The listing builds one solid part. Answer for the finished solid, in the listing's coordinates (mm). Face numbers are marked on the shaded views. A direction names the side the tool comes from. Coordinates: 2 decimals unless noted, no trailing zeros. Order: outer loops, then holes, each group sorted by start corner. A loop starts at its lowest first (then second) coordinate and runs counter-clockwise, first axis right, second up. Notation, with made-up numbers: (-23, 61.25) -> (-15, 61.25) arc R22 ccw to (-15, 94.25) -> close; hole circle Ø8 at (31.25, 19). An arc over 180 degrees is marked (long way). Write each question's results on one line, items separated by ' | '. Start each with the question number.
(1) The part is cut by section B-B, the plane x = -7.5. Give the vertices of the cut face in (y, z), then the cut area to 3 significant figures.
(2) Determine the mould class of the marked faces 6, 7 and 8 for opening direction Z: +Z half, -Z half, draft (parallel to the pull), parting line (faces both ways), or undercut.
(3) A tool of negligible diameter and unlimited length cuts with its end or side. For the marked faces 1, 2, 3, 4 and 5, from which of +Z, -Z, +X, -X, +Y, -Y can it reach the whole face along a straight path? Write none if from no direction.
(4) The part is cut by section C-C, the plane y = 0.55. Give the vertices of the cut face in (x, z).
(5) Given pin 1 (4.5 mm diameter, centred on x = -7.5, z = -11.25, fed in from +Y); pin 2 (2.5 mm diameter, centred on x = -7.5, z = -3.75, fed in from +Y); pin 3 (3 mm diameter, centred on x = -1, z = -8, fed in from -Y); pin 4 (3.5 mm diameter, centred on x = -8.5, z = -5.5, fed in from -Y), each flat-ended and moving along its own axis, determine where each tip first touches the part or whether it passes through.
(6) The part is cut by section D-D, the plane x = -1.25. Give the vertices of the cut face in (y, z), then the cut area to 3 significant figures.
(7) Straight lines are drawn through the part: L1, parallel to Z at x = -0.5, y = 2.15; L2, parallel to X at y = 3.35, z = -7.5; L3, parallel to Z at x = -7, y = 0.5. For each, find the intervals that lie inside material, in ascending order.
(8) The part is cut by section A-A, the plane z = -11.25. Give the vertices of the cut face in (x, y).
```python
from build123d import *

# Parameters (mm, degrees)
SKETCH1_W           = 11
SKETCH1_H           = 15
BOSS_EXTRUDE3_DEPTH = 2
SKETCH2_W           = 4
SKETCH2_H           = 15
BOSS_EXTRUDE4_DEPTH = 2
SKETCH3_W           = 4
SKETCH3_H           = 15
BOSS_EXTRUDE5_DEPTH = 2
SKETCH4_R           = 1.65
CUT_EXTRUDE2_DEPTH  = 13
SKETCH6_W           = 11
SKETCH6_H           = 3
CUT_EXTRUDE4_DEPTH  = 3.8
SKETCH7_R           = 1.5
CUT_EXTRUDE5_DEPTH  = 17.8


with BuildPart() as part:
    # Sketch1 → Boss-Extrude3 (new body)
    with BuildSketch(Plane(origin=(0, 0, 0), x_dir=(1, 0, 0), z_dir=(0, 1, 0))):
        with Locations((-5.5, 7.5)):
            Rectangle(SKETCH1_W, SKETCH1_H)
    extrude(amount=BOSS_EXTRUDE3_DEPTH)

    # Sketch2 → Boss-Extrude4 (add)
    with BuildSketch(Plane(origin=(0, 2, 0), x_dir=(1, 0, 0), z_dir=(0, 1, 0))):
        with Locations((-2, 7.5)):
            Rectangle(SKETCH2_W, SKETCH2_H)
    extrude(amount=BOSS_EXTRUDE4_DEPTH)

    # Sketch3 → Boss-Extrude5 (add)
    with BuildSketch(Plane(origin=(0, 0, 0), x_dir=(-1, 0, 0), z_dir=(0, -1, 0))):
        with Locations((2, 7.5)):
            Rectangle(SKETCH3_W, SKETCH3_H)
    extrude(amount=BOSS_EXTRUDE5_DEPTH)

    # Sketch4 → Cut-Extrude2 (cut)
    with BuildSketch(Plane(origin=(0, 0, 0), x_dir=(-1, 0, 0), z_dir=(0, -1, 0))):
        with Locations(Location((7.5, 11.25, 0), (0, 0, 90))):
            Circle(SKETCH4_R)
        with Locations(Location((7.5, 3.75, 0), (0, 0, 90))):
            Circle(SKETCH4_R)
    extrude(amount=-CUT_EXTRUDE2_DEPTH, mode=Mode.SUBTRACT)

    # Sketch6 → Cut-Extrude4 (cut)
    with BuildSketch(Plane(origin=(0, 0, 0), x_dir=(0, 0, -1), z_dir=(1, 0, 0))):
        with Locations((7.5, 1)):
            Rectangle(SKETCH6_W, SKETCH6_H)
    extrude(amount=-CUT_EXTRUDE4_DEPTH, mode=Mode.SUBTRACT)

    # Sketch7 → Cut-Extrude5 (cut)
    with BuildSketch(Plane(origin=(0, -2, 0), x_dir=(-1, 0, 0), z_dir=(0, -1, 0))):
        with Locations(Location((2, 7.5, 0), (0, 0, 90))):
            Circle(SKETCH7_R)
    extrude(amount=-CUT_EXTRUDE5_DEPTH, mode=Mode.SUBTRACT)


solid = part.part
```
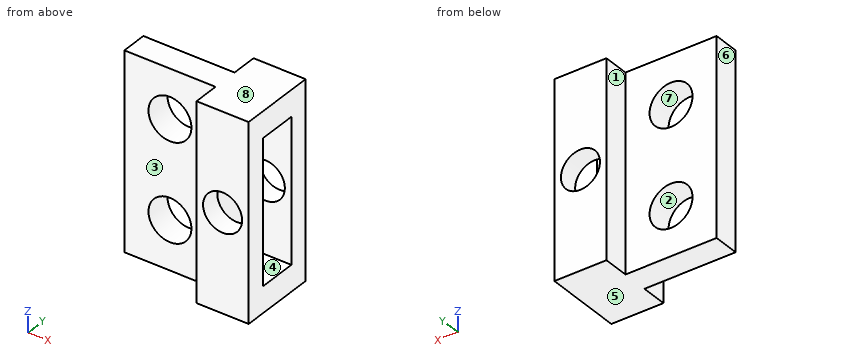
Established:
1) outline: (0, -15) -> (2, -15) -> (2, -12.9) -> (0, -12.9) -> close; (0, -9.6) -> (2, -9.6) -> (2, -5.4) -> (0, -5.4) -> close; (0, -2.1) -> (2, -2.1) -> (2, 0) -> (0, 0) -> close | area: 16.8 mm^2
2) face 6: draft | face 7: undercut | face 8: +Z half
3) face 1: +Z, -Z, -X, +Y | face 2: +Y, -Y | face 3: +Z, -Z, -X, -Y | face 4: +X | face 5: -Z, +X, -X, +Y, -Y
4) outline: (-11, -15) -> (0, -15) -> (0, -13) -> (-3.8, -13) -> (-3.8, -2) -> (0, -2) -> (0, 0) -> (-11, 0) -> close; hole circle Ø3.3 at (-7.5, -11.25); hole circle Ø3.3 at (-7.5, -3.75)
5) pin 1: stops at y = 2 | pin 2: passes through | pin 3: stops at y = -2 | pin 4: stops at y = 0
6) outline: (-2, -15) -> (4, -15) -> (4, -8.8) -> (2.5, -8.8) -> (2.5, -13) -> (-0.5, -13) -> (-0.5, -8.8) -> (-2, -8.8) -> close; (-2, -6.2) -> (-0.5, -6.2) -> (-0.5, -2) -> (2.5, -2) -> (2.5, -6.2) -> (4, -6.2) -> (4, 0) -> (-2, 0) -> close | area: 49.2 mm^2
7) L1: z = -15 to -13, -2 to 0 | L2: x = -4 to -3.5, -0.5 to 0 | L3: z = -15 to -12.82, -9.68 to -5.32, -2.18 to 0
8) outline: (-11, 0) -> (-9.15, 0) -> (-9.15, 2) -> (-11, 2) -> close; (-5.85, 0) -> (-4, 0) -> (-4, -2) -> (0, -2) -> (0, -0.5) -> (-3.8, -0.5) -> (-3.8, 2.5) -> (0, 2.5) -> (0, 4) -> (-4, 4) -> (-4, 2) -> (-5.85, 2) -> close
